from build123d import *

# Parameters (mm, degrees)
BOSS_EXTRUDE1_DEPTH = 1.5
SKETCH4_R           = 2.1
BOSS_EXTRUDE2_DEPTH = 3.5
CUT_EXTRUDE1_DEPTH  = 3.5
CUT_EXTRUDE2_DEPTH  = 51.203735814
BOSS_EXTRUDE3_DEPTH = 1.5


with BuildPart() as part:
    # Sketch2 → Boss-Extrude1 (new body)
    with BuildSketch(Plane.XY):
        Polygon((-41.523066959, 14), (-41.523066959, -14), (6.974355653, -28), (31.223066959, -14), (31.223066959, 14), (6.974355653, 28), align=None)
    extrude(amount=BOSS_EXTRUDE1_DEPTH)

    # Sketch4 → Boss-Extrude2 (add)
    with BuildSketch(Plane.XY.offset(1.5)):
        Polygon((6.974355653, 28), (-41.523066959, 14), (-41.523066959, -14), (6.974355653, -28), (31.223066959, -14), (31.223066959, 14), align=None)
        with Locations((-5.15, 0)):
            Circle(SKETCH4_R, mode=Mode.SUBTRACT)
    extrude(amount=BOSS_EXTRUDE2_DEPTH)

    # Sketch5 → Cut-Extrude1 (cut)
    with BuildSketch(Plane.XY.offset(5)):
        Polygon((-4.477861471, 1.989530045), (-5.822138529, 1.989530045), (-5.822138529, 0.522265885), (-3.115979758, 0.522265885), (3.819278422, 7.561255379), (2.700425446, 7.850425446), (2.408714576, 8.979109263), align=None)
    cut_extrude1 = extrude(amount=-CUT_EXTRUDE1_DEPTH, mode=Mode.SUBTRACT)

    # Sketch9 → Cut-Extrude2 (cut, through all)
    with BuildSketch(Plane.XY.offset(1.5)):
        Polygon((2.408714576, 8.979109263), (2.700425446, 7.850425446), (3.819278422, 7.561255379), (2.009048725, 5.723949904), (0.584447895, 7.127556852), align=None)
    cut_extrude2 = extrude(amount=-CUT_EXTRUDE2_DEPTH, mode=Mode.SUBTRACT)

    # Mirror1: Cut-Extrude1, Cut-Extrude2 across plane
    add(cut_extrude1.mirror(Plane(origin=(0, 0, 0), x_dir=(0, 0, 1), z_dir=(0, -1, 0))), mode=Mode.SUBTRACT)
    add(cut_extrude2.mirror(Plane(origin=(0, 0, 0), x_dir=(0, 0, 1), z_dir=(0, -1, 0))), mode=Mode.SUBTRACT)

    # Sketch8 → Boss-Extrude3 (add)
    with BuildSketch(Plane.XY.offset(1.5)):
        with BuildLine():
            Line((-5.822138529, 0.522265885), (-5.822138529, 1.989530045))
            ThreePointArc((-5.822138529, 1.989530045), (-7.25, 0), (-5.822138529, -1.989530045))
            Line((-5.822138529, -1.989530045), (-5.822138529, -0.522265885))
            Line((-5.822138529, -0.522265885), (-3.115979758, -0.522265885))
            ThreePointArc((-3.115979758, -0.522265885), (-3.05, 0), (-3.115979758, 0.522265885))
            Line((-3.115979758, 0.522265885), (-5.822138529, 0.522265885))
        make_face()
    extrude(amount=BOSS_EXTRUDE3_DEPTH)


solid = part.part
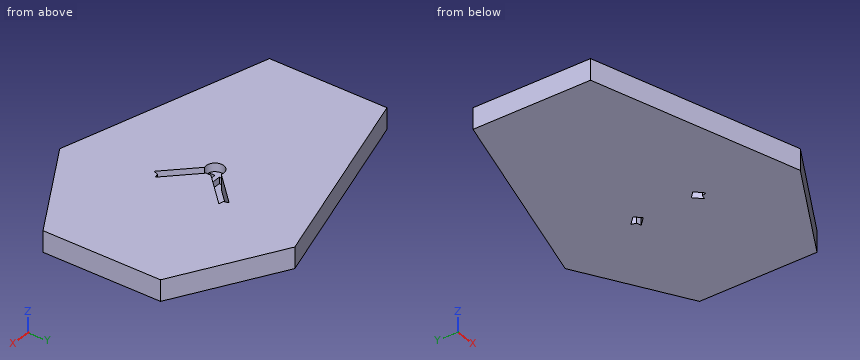
Can you work these out from the model? Positions are in its coordinate system, mm. Round coordinates to 2 decimals unless told otherwise and drop trailing zeros. Write each loop counter-clockwise with the first axis right and the second up, starting at its lowest first coordinate (ties: lowest second). Pieces come first, ordered by that corner, then holes. Notation, with made-up numbers: (-6.5, -0.5) - (23.5, -0.5) arc R20 cw to (23.5, 21.5) - close; hole circle Ø8 at (62.25, -39.75). An arc over 180 degrees is marked (long way). Write each question's results on one line, items separated by ' | '. Start each with the question number.
1) Suppose I cut it at B-B (x = -27). List the corners of the cut face in (y, z) for me, and give its area (3 significant figures).
2) For pin 1 Ø1.6 at (x, z) = (-4, 2.5) entering from +Y; pin 2 Ø3 at (x, z) = (19.5, 3) entering from -Y; pin 3 Ø0.8 at (x, z) = (-4, 2.5) entering from -Y, each with a flat end and sliding along its axis, tell me the tip position at first contact or that it passes through.
3) Suppose I cut it at C-C (y = 24). List the corners of the cut face in (x, z) for me, and give its area (3 significant figures).
4) Please list where these lines run through material, in increasing order: line 1 (X direction, y = 0, z = 3.8); line 2 (Y direction, x = -2, z = 4.6); line 3 (Y direction, x = 3, z = 3.4).
5) Suppose I cut it at A-A (z = 3.75). List the corners of the cut face in (x, y) for me.
Here are the results:
1) outline: (-18.19, 0) - (18.19, 0) - (18.19, 5) - (-18.19, 5) - close | area: 182 mm2
2) pin 1: stops at y = 25.06 | pin 2: stops at y = -21.63 | pin 3: stops at y = -24.95
3) outline: (-6.88, 0) - (13.9, 0) - (13.9, 5) - (-6.88, 5) - close | area: 104 mm2
4) line 1: x = -41.52 to -7.25, -3.05 to 31.22 | line 2: y = -25.41 to -4.5, -1.65 to 1.65, 4.5 to 25.41 | line 3: y = -26.85 to -7.77, -6.73 to 6.73, 7.77 to 26.85
5) outline: (-41.52, -14) - (6.97, -28) - (31.22, -14) - (31.22, 14) - (6.97, 28) - (-41.52, 14) - close; hole (-4.48, -1.99) - (2.41, -8.98) - (2.7, -7.85) - (3.82, -7.56) - (-3.12, -0.52) arc R2.1 ccw to (-3.12, 0.52) - (3.82, 7.56) - (2.7, 7.85) - (2.41, 8.98) - (-4.48, 1.99) arc R2.1 ccw (long way) to start
